Check sheet for the modelled part. Datum: model origin and axes. Units: mm. A direction names the side the tool comes from. Round coordinates to 2 decimals unless told otherwise and drop trailing zeros. Write each loop counter-clockwise with the first axis right and the second up, starting at its lowest first coordinate (ties: lowest second). Pieces come first, ordered by that corner, then holes. Notation, with made-up numbers: (-16, 45.25) -> (-11, 45.25) arc R26 ccw to (-11, 71.25) -> close; hole circle Ø9 at (-31, -10). An arc over 180 degrees is marked (long way). One line per item, written item: value.
from build123d import *

# Parameters (mm, degrees)
SKETCH1_R           = 9.525
BOSS_EXTRUDE1_DEPTH = 5.08
SKETCH2_R           = 6.35
BOSS_EXTRUDE2_DEPTH = 12.7
SKETCH3_R           = 3.175
BOSS_EXTRUDE3_DEPTH = 6.35


with BuildPart() as part:
    # Sketch1 → Boss-Extrude1 (new body)
    with BuildSketch(Plane.XY):
        Circle(SKETCH1_R)
        with BuildLine():
            Line((-1.721227803, 0.894971982), (1.721227803, 0.894971982))
            ThreePointArc((1.721227803, 0.894971982), (0, -1.94), (-1.721227803, 0.894971982))
        make_face(mode=Mode.SUBTRACT)
    extrude(amount=BOSS_EXTRUDE1_DEPTH)

    # Sketch2 → Boss-Extrude2 (add)
    with BuildSketch(Plane(origin=(0, 0, 0), x_dir=(-1, 0, 0), z_dir=(0, 0, -1))):
        with Locations(Location((0, 0, 0), (0, 0, 180))):
            Circle(SKETCH2_R)
    extrude(amount=BOSS_EXTRUDE2_DEPTH)

    # Sketch3 → Boss-Extrude3 (add)
    with BuildSketch(Plane(origin=(0, 0, -12.7), x_dir=(-1, 0, 0), z_dir=(0, 0, -1))):
        Circle(SKETCH3_R)
    extrude(amount=BOSS_EXTRUDE3_DEPTH)


solid = part.part
Item 1: Tool access check on faces 4 (the flat face through (0, 0.895, 3)), 5 (the cylindrical face through (0.69, -3.1, -15.83)), 6 (the flat face through (0, 0, -19.05)). Record the directions out of +Z, -Z, +X, -X, +Y, -Y that give a thin tool (end or side, any length) a straight path to the whole face; none if there is none.
Answer:
face 4: +Z
face 5: -Z
face 6: -Z, +X, -X, +Y, -Y
Item 2: Sectioned sample at D-D on y = 2.5. Enter the section's corners in (x, z), and give its area (3 significant figures).
Answer:
outline: (-9.19, 0) -> (-5.84, 0) -> (-5.84, -12.7) -> (-1.96, -12.7) -> (-1.96, -19.05) -> (1.96, -19.05) -> (1.96, -12.7) -> (5.84, -12.7) -> (5.84, 0) -> (9.19, 0) -> (9.19, 5.08) -> (-9.19, 5.08) -> close
area: 267 mm^2
Item 3: Sectioned sample at C-C on z = -11.75. Enter the section's corners in (x, y), and give its area (3 significant figures).
Answer:
outline: circle Ø12.7 at (0, 0)
area: 127 mm^2
Item 4: Sectioned sample at B-B on x = 0. Enter the section's corners in (y, z) (3 decimals), and give its area (3 significant figures).
Answer:
outline: (-9.525, 0) -> (-6.35, 0) -> (-6.35, -12.7) -> (-3.175, -12.7) -> (-3.175, -19.05) -> (3.175, -19.05) -> (3.175, -12.7) -> (6.35, -12.7) -> (6.35, 0) -> (9.525, 0) -> (9.525, 5.08) -> (0.895, 5.08) -> (0.895, 0) -> (-1.94, 0) -> (-1.94, 5.08) -> (-9.525, 5.08) -> close
area: 284 mm^2
Item 5: Depth check by flat-ended pin: P1, Ø8, axis at x = 3, z = -9.5, coming from the -Y side; P2, Ø3, axis at x = 3.5, z = -3.5, coming from the -Y side; P3, Ø4, axis at x = 7, z = -2.5, coming from the +Y side. Enter the tip coordinate at first touch or a pass-through.
Answer:
P1: stops at y = -6.35
P2: stops at y = -6.03
P3: stops at y = 3.91
Item 6: Mould release check, pull along Y, two halves, no side actions. Record for faces 1 (the cylindrical face through (2.93, 5.634, -6.261)), 2 (the cylindrical face through (0.06, -1.94, 2.5)), 3 (the flat face through (2, -6.2, 0)): pulls with the +Y half, pulls with the -Y half, needs draft (parallel to the pull), parting line crosses it, or undercut.
Answer:
face 1: parting line crosses it
face 2: undercut
face 3: needs draft
Item 7: Thickness scan on line 1 (Y direction, x = 0, z = 2.35) (3 decimals); line 2 (Z direction, x = 4.5, y = -1.5); line 3 (Z direction, x = 4.5, y = 8). Record the ranges inside material, lowest first.
Answer:
line 1: y = -9.525 to -1.94, 0.895 to 9.525
line 2: z = -12.7 to 5.08
line 3: z = 0 to 5.08
Item 8: Sectioned sample at A-A on y = 0. Enter the section's corners in (x, z) (3 decimals), and give its area (3 significant figures).
Answer:
outline: (-9.525, 0) -> (-6.35, 0) -> (-6.35, -12.7) -> (-3.175, -12.7) -> (-3.175, -19.05) -> (3.175, -19.05) -> (3.175, -12.7) -> (6.35, -12.7) -> (6.35, 0) -> (9.525, 0) -> (9.525, 5.08) -> (1.94, 5.08) -> (1.94, 0) -> (-1.94, 0) -> (-1.94, 5.08) -> (-9.525, 5.08) -> close
area: 279 mm^2
